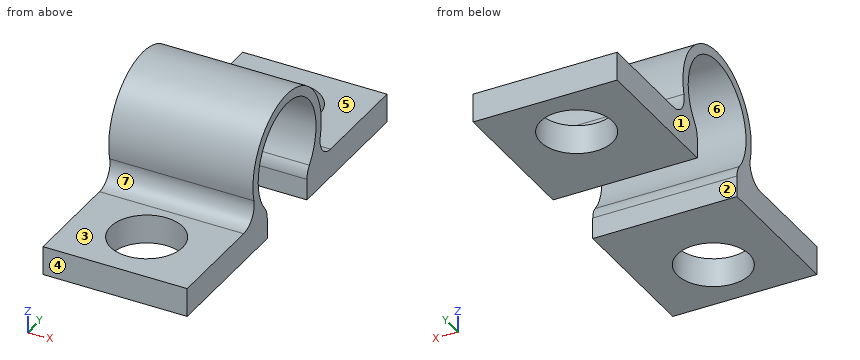
from build123d import *

# Parameters (mm, degrees)
SKETCH1_R           = 3.75
BOSS_EXTRUDE1_DEPTH = 3
SKETCH8_R           = 6.5
SKETCH8_R_2         = 5.5
BOSS_EXTRUDE4_DEPTH = 15
SKETCH9_W           = 15
SKETCH9_H           = 7.549834436
CUT_EXTRUDE5_DEPTH  = 15
FILLET3_R           = 2
FILLET4_R           = 2


with BuildPart() as part:
    # Sketch1 → Boss-Extrude1 (new body)
    with BuildSketch(Plane.XY):
        Polygon((-35.5, -19), (-20.5, -19), (-20.5, 13), (-20.5, 19), (-35.5, 19), align=None)
        with Locations((-28, 13)):
            Circle(SKETCH1_R, mode=Mode.SUBTRACT)
        with Locations((-28, -13)):
            Circle(SKETCH1_R, mode=Mode.SUBTRACT)
    extrude(amount=BOSS_EXTRUDE1_DEPTH)

    # Sketch8 → Boss-Extrude4 (add)
    with BuildSketch(Plane.ZY.offset(35.5)):
        with Locations((7, 0)):
            Circle(SKETCH8_R)
        with Locations((7, 0)):
            Circle(SKETCH8_R_2, mode=Mode.SUBTRACT)
    extrude(amount=-BOSS_EXTRUDE4_DEPTH)

    # Sketch9 → Cut-Extrude5 (cut)
    with BuildSketch(Plane.XY.offset(3)):
        with Locations((-28, 0)):
            Rectangle(SKETCH9_W, SKETCH9_H)
    extrude(amount=-CUT_EXTRUDE5_DEPTH, mode=Mode.SUBTRACT)

    # Fillet3
    fillet3_edges = [part.edges().sort_by_distance(p)[0] for p in [
        (-28, -5.123475383, 3),
        (-28, 5.123475383, 3),
    ]]
    fillet(fillet3_edges, radius=FILLET3_R)

    # Fillet4
    fillet4_edges = [part.edges().sort_by_distance(p)[0] for p in [
        (-28, -3.774917218, 3),
        (-28, 3.774917218, 3),
    ]]
    fillet(fillet4_edges, radius=FILLET4_R)


solid = part.part
CAD build for the part. Positions are in the model's coordinates, mm. Face numbers are marked on the shaded views. A direction names the side the tool comes from. Round coordinates to 2 decimals unless told otherwise and drop trailing zeros. Order: outer loops, then holes, each group sorted by start corner. A loop starts at its lowest first (then second) coordinate and runs counter-clockwise, first axis right, second up. Notation, with made-up numbers: M 42,-14 L 78,-14 A28 ccw 78,21 Z; hole C -37,78.25 d3. An arc over 180 degrees is marked long. Use one line per item in the form item = value.
Q1. Two-plate mould, pull along Z, no slides. Class the marked faces 4, 5, 6 and 7: +Z half, -Z half, draft (parallel to the pull), parting line (faces both ways), or undercut.
Recorded:
face_4 = draft
face_5 = +Z half
face_6 = undercut
face_7 = undercut
Q2. Probe L1, parallel to Y at x = -28, z = 1.45; L2, parallel to Y at x = -30.25, z = 7; L3, parallel to Z at x = -29, y = 0. List the from-to ranges inside material, lowest first.
Recorded:
L1 = -19 to -16.75, -9.25 to -3.77, 3.77 to 9.25, 16.75 to 19
L2 = -6.5 to -5.5, 5.5 to 6.5
L3 = 12.5 to 13.5
Q3. Saw through at B-B on z = 10.75. Give the cut face in (x, y), then the cut area to 3 significant figures.
Recorded:
outline = M -35.5,-5.31 L -20.5,-5.31 L -20.5,-4.02 L -35.5,-4.02 Z; M -35.5,4.02 L -20.5,4.02 L -20.5,5.31 L -35.5,5.31 Z
area = 38.6 mm^2
Q4. Saw through at D-D on x = -22.5. Give the cut face in (y, z), then the cut area to 3 significant figures.
Recorded:
outline = M -19,0 L -3.77,0 L -3.77,2.21 A2 ccw -4.23,3.49 A5.5 cw long 4.23,3.49 A2 ccw 3.77,2.21 L 3.77,0 L 19,0 L 19,3 L 8.26,3 A2 cw 6.32,5.47 A6.5 ccw long -6.32,5.47 A2 cw -8.26,3 L -19,3 Z
area = 123 mm^2
Q5. Flat gauge pins, fed straight in: P1, Ø3, axis at x = -25, y = 11, coming from the +Z side; P2, Ø1, axis at x = -33, y = -1.5, coming from the +Z side. Where does each tip first touch, or does it go through?
Recorded:
P1 = 3
P2 = 13.42
Q6. Saw through at C-C on x = -26.75. Give the cut face in (y, z), then the cut area to 3 significant figures.
Recorded:
outline = M -19,0 L -16.54,0 L -16.54,3 L -19,3 Z; M -9.46,0 L -3.77,0 L -3.77,2.21 A2 ccw -4.23,3.49 A5.5 cw long 4.23,3.49 A2 ccw 3.77,2.21 L 3.77,0 L 9.46,0 L 9.46,3 L 8.26,3 A2 cw 6.32,5.47 A6.5 ccw long -6.32,5.47 A2 cw -8.26,3 L -9.46,3 Z; M 16.54,0 L 19,0 L 19,3 L 16.54,3 Z
area = 80.3 mm^2
Q7. Saw through at A-A on y = -13. Give the cut face in (x, z), then the cut area to 3 significant figures.
Recorded:
outline = M -35.5,0 L -31.75,0 L -31.75,3 L -35.5,3 Z; M -24.25,0 L -20.5,0 L -20.5,3 L -24.25,3 Z
area = 22.5 mm^2
Q8. Which spindle directions (+Z, -Z, +X, -X, +Y, -Y) get a long thin tool onto all of the face, cutting with end or side? Do the marked faces 1, 2 and 3. Say none if no direction does.
Recorded:
face_1 = +Z, -Z, -X, +Y, -Y
face_2 = -Z, +X, -X
face_3 = +Z, +X, -X, -Y
